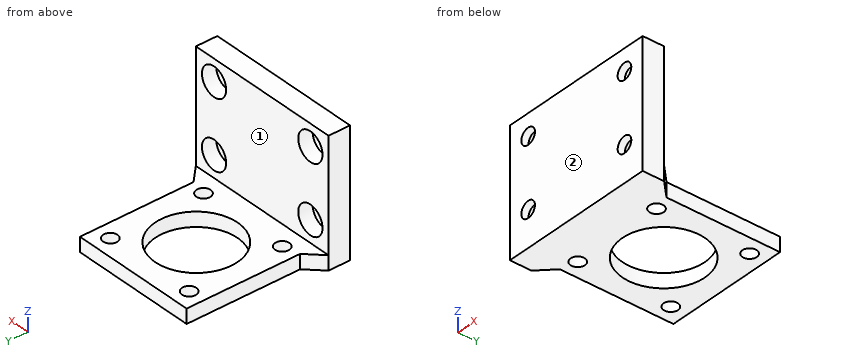
Autodesk Inventor part; units mm, degrees
ref_plane "YZ Plane" through (0, 0, 0) normal (1, 0, 0) x (0, 1, 0)
ref_plane "XZ Plane" through (0, 0, 0) normal (0, 1, 0) x (-1, 0, 0)
ref_plane "XY Plane" through (0, 0, 0) normal (0, 0, 1) x (1, 0, 0)
sketch "Sketch1" plane through (0, 0, 0) normal (0, 1, 0) x (-1, 0, 0)
  circle A0 centre (15.9, 35) radius 2.25
  circle A1 centre (15.9, 16) radius 2.25
  circle A2 centre (-15.9, 16) radius 2.25
  circle A3 centre (-15.9, 35) radius 2.25
  line L0 (21.9, 10) -> (-21.9, 10)
  line L1 (-21.9, 10) -> (-21.9, 41)
  line L2 (-21.9, 41) -> (21.9, 41)
  line L3 (21.9, 41) -> (21.9, 10)
  point P0 (0, 0)
  point P1 (0, 0)
  dimension "d0" = 43.8
  dimension "d1" = 31
extrude "Extrusion1" add sketch "Sketch1" along normal blind 6
sketch "Sketch2" plane through (0, 6, 0) normal (0, 1, 0) x (1, 0, 0)
  circle A0 centre (-15.9, -16) radius 2.25
  circle A1 centre (-15.9, -16) radius 4
  circle A2 centre (-15.9, -35) radius 2.25
  circle A3 centre (-15.9, -35) radius 4
  circle A4 centre (15.9, -35) radius 2.25
  circle A5 centre (15.9, -35) radius 4
  circle A6 centre (15.9, -16) radius 2.25
  circle A7 centre (15.9, -16) radius 4
  point P0 (0, 0)
  dimension "d4" = 8
  dimension "d5" = 8
  dimension "d6" = 8
  dimension "d7" = 8
extrude "Extrusion2" cut sketch "Sketch2" against normal blind 4
sketch "Sketch3" plane through (21.9, 0, 10) normal (0, 0, -1) x (-1, 0, 0)
  line L0 (43.8, 0) -> (0, 0)
  line L1 (43.8, 0) -> (43.8, 6)
  line L2 (0, 6) -> (43.8, 6)
  line L3 (0, 0) -> (0, 6)
  line L4 (43.8, 6) -> (0, 6)
  line L5 (21.9, 6) -> (39.5, 6)
  line L6 (39.5, 6) -> (39.5, 42)
  line L7 (39.5, 42) -> (21.9, 42)
  line L8 (39.5, 42) -> (4.3, 42)
  line L9 (4.3, 42) -> (4.3, 6)
  line L10 (4.3, 6) -> (39.5, 6)
  line L11 (39.5, 6.8) -> (39.5, 42)
  circle A0 centre (34.9, 37.4) radius 2
  circle A1 centre (8.9, 37.4) radius 2
  circle A2 centre (8.9, 11.4) radius 2
  circle A3 centre (34.9, 11.4) radius 2
  circle A4 centre (21.9, 24.4) radius 11.5
  point P0 (21.9, 0)
  dimension "d16" = 4
  dimension "d19" = 360
  dimension "d21" = 23
extrude "Extrusion3" add sketch "Sketch3" along normal blind 4
chamfer "Chamfer1" distance 4.3 angle 45 1 edges at (17.6, 6, 8)
chamfer "Chamfer2" distance 4.3 angle 45 1 edges at (-17.6, 6, 8)
properties part number "NEMA14 Mounting Bracket"
The model under review builds one solid part; all positions refer to its coordinate system, in mm. Face numbers are marked on the shaded views. A direction names the side the tool comes from. Coordinates: 2 decimals unless noted, no trailing zeros. Write each loop counter-clockwise with the first axis right and the second up, starting at its lowest first coordinate (ties: lowest second). Pieces come first, ordered by that corner, then holes.
1) We need section C-C on x = 0. State the section outline as (y, z) points.
2) Machinability: for the marked faces 1 and 2, which of the approach directions +Z, -Z, +X, -X, +Y, -Y give a long, thin tool a straight path to every point of the face, cutting with its end or side? Answer none if there is none.
3) We need section D-D on z = 16. State the section outline as (x, y) points.
4) We need section A-A on x = -15.9. State the section outline as (y, z) points, then the cut area to 3 significant figures.
5) Clearance check with flat-ended pins moving along their axes: pin 1 Ø10.5 at (x, z) = (-15.9, 16) entering from +Y; pin 2 Ø2 at (y, z) = (27, 7.5) entering from +X; pin 3 Ø4 at (x, z) = (-15, 16.5) entering from +Y. State where each tip first meets the part, or that it passes through.
6) To check wall thickness, follow probe 1 along Z at (x, y) = (-15.9, 3.35); probe 2 along Y at (x, z) = (13, 8); probe 3 along X at (y, z) = (4.95, 16). State the ranges of each line that lie inside material, in increasing order.
7) We need section B-B on y = 37.4. State the section outline as (x, z) points, then the cut area to 3 significant figures.
Answer list:
1. outline: (0, 6) - (12.9, 6) - (12.9, 10) - (6, 10) - (6, 41) - (0, 41) - close; (35.9, 6) - (42, 6) - (42, 10) - (35.9, 10) - close
2. face 1: +Z, +X, -X, +Y
2. face 2: +Z, -Z, +X, -X, -Y
3. outline: (-21.9, 0) - (-18.15, 0) - (-18.15, 2) - (-19.9, 2) - (-19.9, 6) - (-21.9, 6) - close; (-13.65, 0) - (13.65, 0) - (13.65, 2) - (11.9, 2) - (11.9, 6) - (-11.9, 6) - (-11.9, 2) - (-13.65, 2) - close; (18.15, 0) - (21.9, 0) - (21.9, 6) - (19.9, 6) - (19.9, 2) - (18.15, 2) - close
4. outline: (0, 6) - (42, 6) - (42, 10) - (6, 10) - (6, 12) - (2, 12) - (2, 13.75) - (0, 13.75) - close; (0, 18.25) - (2, 18.25) - (2, 20) - (6, 20) - (6, 31) - (2, 31) - (2, 32.75) - (0, 32.75) - close; (0, 37.25) - (2, 37.25) - (2, 39) - (6, 39) - (6, 41) - (0, 41) - close
4. area: 272 mm2
5. pin 1: stops at y = 6
5. pin 2: stops at x = 17.6
5. pin 3: stops at y = 2
6. probe 1: z = 6 to 12, 20 to 31, 39 to 41
6. probe 2: y = 0 to 9.4, 13.4 to 35.4, 39.4 to 42
6. probe 3: x = -21.9 to -19.9, -11.9 to 11.9, 19.9 to 21.9
7. outline: (-17.6, 6) - (-15, 6) - (-15, 10) - (-17.6, 10) - close; (-11, 6) - (11, 6) - (11, 10) - (-11, 10) - close; (15, 6) - (17.6, 6) - (17.6, 10) - (15, 10) - close
7. area: 109 mm2
